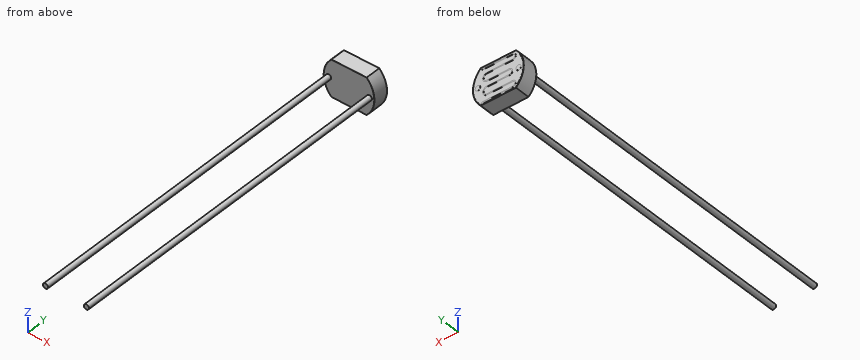
from build123d import *
from build123d.topology import SkipClean

# Parameters (mm, degrees)
BOSS_EXTRUDE1_DEPTH      = 1.5
BOSS_EXTRUDE2_DEPTH      = 0.01
BOSS_EXTRUDE3_DEPTH      = 0.01
BOSS_EXTRUDE4_DEPTH      = 0.01
BOSS_EXTRUDE4_DEPTH_BACK = 35
SKETCH4_R                = 0.25
FILLET1_R                = 0.01


with BuildPart() as part:
    # Sketch1 → Boss-Extrude1 (new body)
    with BuildSketch(Plane(origin=(0, 0, 0), x_dir=(1, 0, 0), z_dir=(0, 1, 0))):
        with BuildLine():
            Line((-1.734935157, 1.8), (1.734935157, 1.8))
            ThreePointArc((1.734935157, 1.8), (2.5, 0), (1.734935157, -1.8))
            Line((1.734935157, -1.8), (-1.734935157, -1.8))
            ThreePointArc((-1.734935157, -1.8), (-2.5, 0), (-1.734935157, 1.8))
        make_face()
    extrude(amount=BOSS_EXTRUDE1_DEPTH)

    # Sketch2 → Boss-Extrude2 (add)
    with BuildSketch(Plane(origin=(0, 1.5, 0), x_dir=(1, 0, 0), z_dir=(0, 1, 0))):
        with BuildLine():
            Line((-1.71464282, -1.75), (1.71464282, -1.75))
            ThreePointArc((1.71464282, -1.75), (2.45, 0), (1.71464282, 1.75))
            Line((1.71464282, 1.75), (-1.71464282, 1.75))
            ThreePointArc((-1.71464282, 1.75), (-2.45, 0), (-1.71464282, -1.75))
        make_face()
    extrude(amount=BOSS_EXTRUDE2_DEPTH)

    # Sketch3 → Boss-Extrude3 (add)
    with SkipClean():  # the faces are left unmerged after this step: merging them gives an invalid solid
        with BuildSketch(Plane(origin=(0, 1.51, 0), x_dir=(1, 0, 0), z_dir=(0, 1, 0))):
            with BuildLine():
                Line((-1.100223992, 0.325), (1.100223992, 0.325))
                ThreePointArc((1.100223992, 0.325), (1.425223992, 0.65), (1.100223992, 0.975))
                Line((1.100223992, 0.975), (-1.100223992, 0.975))
                Line((-1.100223992, 0.975), (-1.415621536, 0.975))
                ThreePointArc((-1.415621536, 0.975), (-1.740621536, 1.3), (-1.415621536, 1.625))
                Line((-1.415621536, 1.625), (1.100223992, 1.625))
                Line((1.100223992, 1.625), (1.414873992, 1.625))
                ThreePointArc((1.414873992, 1.625), (1.55739592, 1.657916964), (1.671047761, 1.75))
                Line((1.671047761, 1.75), (1.71464282, 1.75))
                ThreePointArc((1.71464282, 1.75), (1.737970537, 1.726834796), (1.760985316, 1.703358658))
                ThreePointArc((1.760985316, 1.703358658), (1.609556335, 1.572211984), (1.414873992, 1.525))
                Line((1.414873992, 1.525), (1.100223992, 1.525))
                Line((1.100223992, 1.525), (-1.415621536, 1.525))
                ThreePointArc((-1.415621536, 1.525), (-1.640621536, 1.3), (-1.415621536, 1.075))
                Line((-1.415621536, 1.075), (-1.100223992, 1.075))
                Line((-1.100223992, 1.075), (1.100223992, 1.075))
                ThreePointArc((1.100223992, 1.075), (1.525223992, 0.65), (1.100223992, 0.225))
                Line((1.100223992, 0.225), (-1.100223992, 0.225))
                ThreePointArc((-1.100223992, 0.225), (-1.325223992, 0), (-1.100223992, -0.225))
                Line((-1.100223992, -0.225), (1.100223992, -0.225))
                ThreePointArc((1.100223992, -0.225), (1.525223992, -0.65), (1.100223992, -1.075))
                Line((1.100223992, -1.075), (-1.100223992, -1.075))
                Line((-1.100223992, -1.075), (-1.415621536, -1.075))
                ThreePointArc((-1.415621536, -1.075), (-1.640621536, -1.3), (-1.415621536, -1.525))
                Line((-1.415621536, -1.525), (1.100223992, -1.525))
                Line((1.100223992, -1.525), (1.414873992, -1.525))
                ThreePointArc((1.414873992, -1.525), (1.609556335, -1.572211984), (1.760985316, -1.703358658))
                ThreePointArc((1.760985316, -1.703358658), (1.737970537, -1.726834796), (1.71464282, -1.75))
                Line((1.71464282, -1.75), (1.671047761, -1.75))
                ThreePointArc((1.671047761, -1.75), (1.55739592, -1.657916964), (1.414873992, -1.625))
                Line((1.414873992, -1.625), (1.100223992, -1.625))
                Line((1.100223992, -1.625), (-1.415621536, -1.625))
                ThreePointArc((-1.415621536, -1.625), (-1.740621536, -1.3), (-1.415621536, -0.975))
                Line((-1.415621536, -0.975), (-1.100223992, -0.975))
                Line((-1.100223992, -0.975), (1.100223992, -0.975))
                ThreePointArc((1.100223992, -0.975), (1.425223992, -0.65), (1.100223992, -0.325))
                Line((1.100223992, -0.325), (-1.100223992, -0.325))
                ThreePointArc((-1.100223992, -0.325), (-1.425223992, 0), (-1.100223992, 0.325))
            make_face()
        extrude(amount=BOSS_EXTRUDE3_DEPTH)

    # Sketch4 → Boss-Extrude4 (add, two sides: drawn at the far end of the back side and taken through both)
    with SkipClean():  # the faces are left unmerged after this step: merging them gives an invalid solid
        with BuildSketch(Plane(origin=(0, 1.51, 0), x_dir=(1, 0, 0), z_dir=(0, 1, 0)).offset(-BOSS_EXTRUDE4_DEPTH_BACK)):
            with Locations(Location((-2.009742492, 0, 0), (0, 0, 270))):
                Circle(SKETCH4_R)
            with Locations(Location((2.009742492, 0, 0), (0, 0, 270))):
                Circle(SKETCH4_R)
        extrude(amount=BOSS_EXTRUDE4_DEPTH + BOSS_EXTRUDE4_DEPTH_BACK)

    # Fillet1
    fillet1_edges = [part.edges().sort_by_distance(p)[0] for p in [
        (2.5, 1.5, 0),
        (0, 1.5, -1.8),
        (-2.5, 1.5, 0),
        (0, 0, -1.8),
        (2.5, 0, 0),
        (0, 0, 1.8),
        (-2.5, 0, 0),
        (0, 1.5, 1.8),
        (1.734935157, 0.75, -1.8),
        (1.734935157, 0.75, 1.8),
        (-1.734935157, 0.75, 1.8),
    ]]
    fillet(fillet1_edges, radius=FILLET1_R)


solid = part.part
Build history of the part. All positions in model axes, mm. Give positions to 0.01 mm unless a question says otherwise; leave off trailing zeros. Order: outer loops, then holes, each group sorted by start corner. A loop starts at its lowest first (then second) coordinate and runs counter-clockwise, first axis right, second up. Notation, with made-up numbers: M 17,26.25 L 39,26.25 A24 ccw 39,43.25 Z; hole C 77,-24 d10. An arc over 180 degrees is marked long. Use one line per item in the form item = value.
Q1. Slice it at A-A, the plane y = -7. Write the cut outline in (x, z).
Conclusion:
outline = C -2.01,0 d0.5; C 2.01,0 d0.5
Q2. Wall check: probe 1 along Y at (x, z) = (1.8, -1.2); probe 2 along X at (y, z) = (-25, 0.1); probe 3 along Z at (x, y) = (2.2, -22). Give the ranges that are in metal, low to high.
Conclusion:
probe_1 = 0 to 1.51
probe_2 = -2.24 to -1.78, 1.78 to 2.24
probe_3 = -0.16 to 0.16
Q3. Pin check, flat tips, straight feed: P1, Ø2, axis at y = -8.5, z = -0.5, coming from the -X side; P2, Ø1, axis at x = 2, z = -1, coming from the +Y side; P3, Ø1, axis at x = 1, z = -1.5, coming from the -Y side. Stop position of each tip, or through.
Conclusion:
P1 = -2.26
P2 = 1.51
P3 = 0
